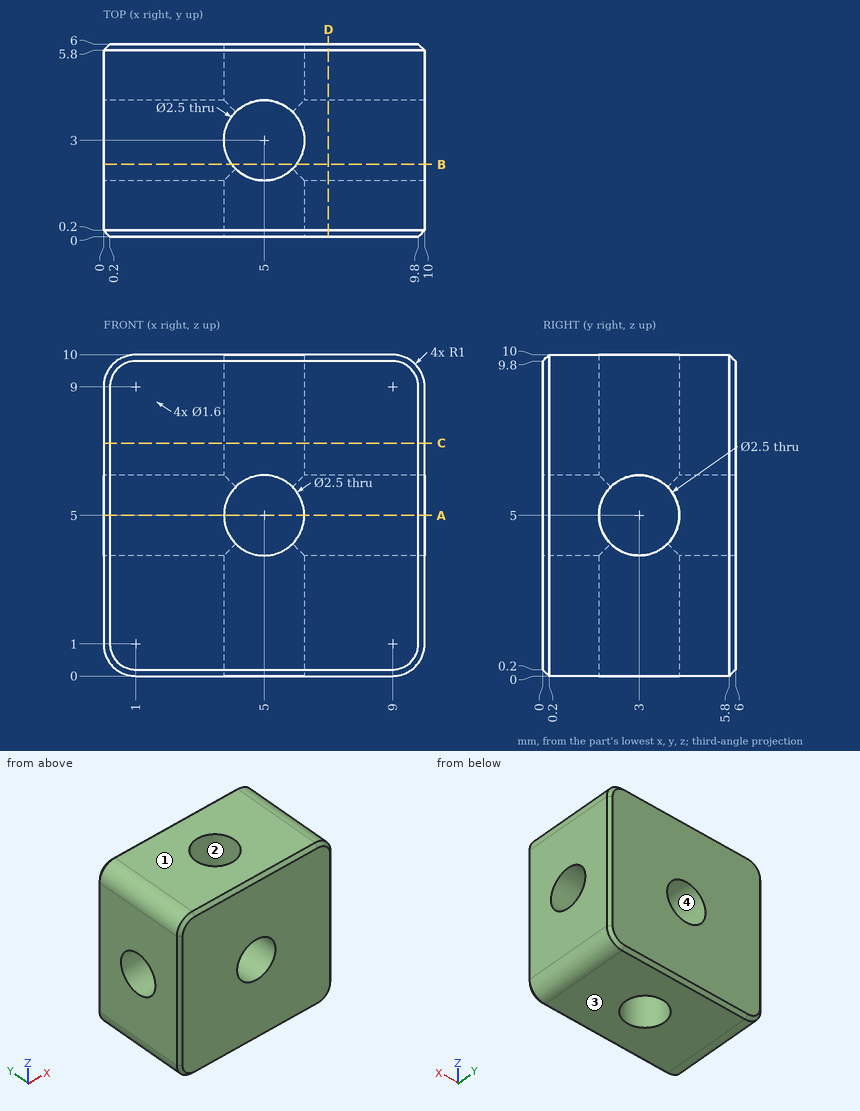
Answer from the drawing. Dimensions are ordinates in mm from the lowest x, y and z of the part. Coordinates: 2 decimals unless noted, no trailing zeros. Loops run counter-clockwise (first coordinate to the right, second up) from the corner with the lowest first, then second, coordinate; pieces in that order, holes last. Notation, with made-up numbers: (30.25, 62) -> (87.25, 62) arc R11 ccw to (87.25, 78) -> close; hole circle Ø2 at (50.25, 49). An arc over 180 degrees is marked (long way). Return JSON: item names as keys, results as strings.
Item 1: Find the intervals of material crossed by probe 1 along Y at (x, z) = (2.6, 5); probe 2 along X at (y, z) = (3, 7.9); probe 3 along Z at (x, y) = (6.5, 3.25), in increasing order.
Answers:
{"probe 1": "y = 0 to 1.75, 4.25 to 6", "probe 2": "x = 0 to 3.75, 6.25 to 10", "probe 3": "z = 0 to 3.78, 6.22 to 10"}
Item 2: Find section B-B (y = 2.25). Determine the outline of the cut face in (x, z).
Answers:
{"outline": "(0, 1) arc R1 ccw to (1, 0) -> (4, 0) -> (4, 4) -> (0, 4) -> close; (0, 6) -> (4, 6) -> (4, 10) -> (1, 10) arc R1 ccw to (0, 9) -> close; (6, 0) -> (9, 0) arc R1 ccw to (10, 1) -> (10, 4) -> (6, 4) -> close; (6, 6) -> (10, 6) -> (10, 9) arc R1 ccw to (9, 10) -> (6, 10) -> close"}
Item 3: Find section A-A (z = 5). Determine the outline of the cut face in (x, y).
Answers:
{"outline": "(0, 0.2) -> (0.2, 0) -> (3.75, 0) -> (3.75, 1.75) -> (0, 1.75) -> close; (0, 4.25) -> (3.75, 4.25) -> (3.75, 6) -> (0.2, 6) -> (0, 5.8) -> close; (6.25, 0) -> (9.8, 0) -> (10, 0.2) -> (10, 1.75) -> (6.25, 1.75) -> close; (6.25, 4.25) -> (10, 4.25) -> (10, 5.8) -> (9.8, 6) -> (6.25, 6) -> close"}
Item 4: Find section D-D (x = 7). Determine the outline of the cut face in (y, z), plus the area to 3 significant figures.
Answers:
{"outline": "(0, 0.2) -> (0.2, 0) -> (5.8, 0) -> (6, 0.2) -> (6, 9.8) -> (5.8, 10) -> (0.2, 10) -> (0, 9.8) -> close; hole circle Ø2.5 at (3, 5)", "area": "55.0 mm2"}
Item 5: Flat-ended cylindrical pins translate along their axes: P1, Ø3, axis at x = 5, y = 3, coming from the -Z side; P2, Ø2, axis at y = 3, z = 5, coming from the -X side. Find the tip coordinate at first contact, or state that the pin passes through.
Answers:
{"P1": "stops at z = 0", "P2": "passes through"}
Item 6: Find section C-C (z = 7.25). Determine the outline of the cut face in (x, y), plus the area to 3 significant figures.
Answers:
{"outline": "(0, 0.2) -> (0.2, 0) -> (9.8, 0) -> (10, 0.2) -> (10, 5.8) -> (9.8, 6) -> (0.2, 6) -> (0, 5.8) -> close; hole circle Ø2.5 at (5, 3)", "area": "55.0 mm2"}
Item 7: For a pull along Z with two mould halves and no side action, classify the marked faces 1, 2, 3 and 4 as +Z half, -Z half, draft (parallel to the pull), parting line (faces both ways), or undercut.
Answers:
{"face 1": "+Z half", "face 2": "draft", "face 3": "-Z half", "face 4": "undercut"}
